Autodesk Inventor part; units mm, degrees
ref_plane "YZ Plane" through (0, 0, 0) normal (1, 0, 0) x (0, 1, 0)
ref_plane "XZ Plane" through (0, 0, 0) normal (0, 1, 0) x (-1, 0, 0)
ref_plane "XY Plane" through (0, 0, 0) normal (0, 0, 1) x (1, 0, 0)
sketch "Sketch1" plane through (0, 0, 0) normal (0, 1, 0) x (-1, 0, 0)
  line L0 (-83.5, 139.5) -> (83.5, 139.5)
  line L1 (83.5, 139.5) -> (83.5, -139.5)
  line L2 (83.5, -139.5) -> (-83.5, -139.5)
  line L3 (-83.5, -139.5) -> (-83.5, 139.5)
  line L4 (-83.5, 139.5) -> (83.5, -139.5) construction
  line L5 (83.5, 139.5) -> (-83.5, -139.5) construction
  point P0 (0, 0)
  dimension "d0" = 167
  dimension "d1" = 279
extrude "Extrusion1" add sketch "Sketch1" along normal blind 26.6
sketch "Sketch2" plane through (0, 26.6, 0) normal (0, 1, 0) x (1, 0, 0)
  line L0 (71.5, -119.5) -> (-71.5, -119.5)
  line L1 (-73.5, -117.5) -> (-73.5, 117.5)
  line L2 (-71.5, 119.5) -> (71.5, 119.5)
  line L3 (73.5, 117.5) -> (73.5, -117.5)
  line L4 (73.5, -119.5) -> (-73.5, 119.5) construction
  line L5 (-73.5, -119.5) -> (73.5, 119.5) construction
  arc A0 (-73.5, -117.5) -> (-71.5, -119.5) centre (-71.5, -117.5) ccw
  arc A1 (-71.5, 119.5) -> (-73.5, 117.5) centre (-71.5, 117.5) ccw
  arc A2 (73.5, 117.5) -> (71.5, 119.5) centre (71.5, 117.5) ccw
  arc A3 (71.5, -119.5) -> (73.5, -117.5) centre (71.5, -117.5) ccw
  point P0 (0, 0)
  dimension "d4" = 147
  dimension "d5" = 239
  dimension "d6" = 2
extrude "Extrusion2" cut sketch "Sketch2" against normal blind 1.1
sketch "Sketch3" plane through (0, 25.5, 0) normal (0, 1, 0) x (1, 0, 0)
  line L0 (-73.5, -117.5) -> (-73.5, 117.5)
  line L1 (71.5, -119.5) -> (-71.5, -119.5)
  line L2 (-72.25, -117.83) -> (72.25, -117.83)
  line L3 (72.25, -117.83) -> (72.25, 112.27)
  line L4 (72.25, 112.27) -> (-72.25, 112.27)
  line L5 (-72.25, 112.27) -> (-72.25, -117.83)
  point P0 (0, 0)
  dimension "d9" = 1.25
  dimension "d10" = 1.67
  dimension "d11" = 144.5
  dimension "d12" = 230.1
extrude "Extrusion3" cut sketch "Sketch3" against normal blind 20
sketch "Sketch4" plane through (0, 5.5, 0) normal (0, 1, 0) x (1, 0, 0)
  circle A0 centre (-66.5, -111.83) radius 2
  line L0 (72.25, -117.83) -> (-72.25, -117.83)
  line L1 (-72.25, -117.83) -> (-72.25, 112.27)
  circle A1 centre (66.5, -111.83) radius 2
  line L2 (72.25, 112.27) -> (72.25, -117.83)
  circle A2 centre (-66.5, 106.27) radius 2
  line L3 (-72.25, 112.27) -> (72.25, 112.27)
  circle A3 centre (66.5, 106.27) radius 2
  point P0 (0, 0)
  dimension "d15" = 4
  dimension "d16" = 6
  dimension "d17" = 5.75
  dimension "d18" = 4
  dimension "d19" = 6
  dimension "d20" = 5.75
  dimension "d21" = 4
  dimension "d22" = 5.75
  dimension "d23" = 6
  dimension "d24" = 4
  dimension "d25" = 6
  dimension "d26" = 5.75
extrude "Extrusion4" add sketch "Sketch4" along normal blind 10.3 contours A0 | A1 | A2 | A3
sketch "Sketch5" plane through (0, 5.5, 0) normal (0, 1, 0) x (1, 0, 0)
  circle A0 centre (-66.5, -111.83) radius 2
  circle A1 centre (-66.5, -111.83) radius 1.25
  circle A2 centre (-66.5, 106.27) radius 2
  circle A3 centre (-66.5, 106.27) radius 1.25
  circle A4 centre (66.5, 106.27) radius 2
  circle A5 centre (66.5, 106.27) radius 1.25
  circle A6 centre (66.5, -111.83) radius 1.25
  point P0 (0, 0)
  dimension "d29" = 2.5
  dimension "d30" = 2.5
  dimension "d31" = 2.5
  dimension "d32" = 2.5
extrude "Extrusion5" cut sketch "Sketch5" along normal blind 10.3 and the other way blind 5.5 contours A1 | A3 | A5 | A6
sketch "Sketch8" plane through (0, 0, 0) normal (0, -1, 0) x (1, 0, 0)
  circle A0 centre (66.5, 111.83) radius 1.25
  circle A1 centre (66.5, 111.83) radius 1.75
  circle A2 centre (66.5, -106.27) radius 1.25
  circle A3 centre (66.5, -106.27) radius 1.75
  circle A4 centre (-66.5, -106.27) radius 1.25
  circle A5 centre (-66.5, -106.27) radius 1.75
  circle A6 centre (-66.5, 111.83) radius 1.75
  point P0 (0, 0)
  dimension "d49" = 3.5
  dimension "d50" = 3.5
  dimension "d51" = 3.5
  dimension "d52" = 3.5
extrude "Extrusion8" cut sketch "Sketch8" against normal blind 13.8
sketch "Sketch9" plane through (0, 5.5, 0) normal (0, 1, 0) x (1, 0, 0)
  line L0 (60, -100) -> (-60, -100)
  line L1 (-60, -100) -> (-60, 100)
  line L2 (-60, 100) -> (60, 100)
  line L3 (60, 100) -> (60, -100)
  line L4 (60, -100) -> (-60, 100) construction
  line L5 (-60, -100) -> (60, 100) construction
  point P0 (0, 0)
  dimension "d55" = 120
  dimension "d56" = 200
extrude "Extrusion9" cut sketch "Sketch9" against normal blind 5.8
sketch "Sketch10" plane through (0, 0, 0) normal (0, -1, 0) x (1, 0, 0)
  line L0 (83.5, 139.5) -> (83.5, -139.5)
  line L1 (-83.5, -139.5) -> (-83.5, 139.5)
  line L2 (83.5, 139.5) -> (-83.5, 139.5)
  line L3 (-83.5, 139.5) -> (-83.5, -139.5)
  line L4 (-83.5, -139.5) -> (83.5, -139.5)
  line L5 (83.5, -139.5) -> (83.5, 139.5)
  line L6 (72.25, -115.05) -> (-72.25, -115.05)
  line L7 (-72.25, -115.05) -> (-72.25, 115.05)
  line L8 (-72.25, 115.05) -> (72.25, 115.05)
  line L9 (72.25, 115.05) -> (72.25, -115.05)
  line L10 (72.25, -115.05) -> (-72.25, 115.05) construction
  line L11 (-72.25, -115.05) -> (72.25, 115.05) construction
  line L12 (-83.5, -139.5) -> (83.5, -139.5)
  line L13 (83.5, -139.5) -> (83.5, 139.5)
  line L14 (83.5, 139.5) -> (-83.5, 139.5)
  line L15 (-83.5, 139.5) -> (-83.5, -139.5)
  point P0 (0, 0)
  point P1 (71.5, 119.5)
  dimension "d67" = 144.5
  dimension "d68" = 230.1
extrude "Extrusion10" add sketch "Sketch10" along normal blind 40
sketch "Sketch12" plane through (0, -40, 0) normal (0, -1, 0) x (1, 0, 0)
  line L0 (-72.25, -115.05) -> (-72.25, 115.05)
  line L1 (72.25, -115.05) -> (-72.25, -115.05)
  line L2 (-77.25, -120.05) -> (-72.25, -120.05)
  line L3 (-72.25, -120.05) -> (-72.25, 120.05)
  line L4 (-72.25, 120.05) -> (-77.25, 120.05)
  line L5 (-77.25, 120.05) -> (-77.25, -120.05)
  line L6 (72.25, 115.05) -> (72.25, -115.05)
  line L7 (77.25, -120.05) -> (72.25, -120.05)
  line L8 (72.25, -120.05) -> (72.25, 120.05)
  line L9 (72.25, 120.05) -> (77.25, 120.05)
  line L10 (77.25, 120.05) -> (77.25, -120.05)
  line L11 (72.25, 115.05) -> (-72.25, 115.05)
  line L12 (72.25, 120.05) -> (-72.25, 120.05)
  line L13 (-72.25, 120.05) -> (-72.25, 115.05)
  line L14 (-72.25, 115.05) -> (72.25, 115.05)
  line L15 (72.25, 115.05) -> (72.25, 120.05)
  line L16 (-83.5, 139.5) -> (-83.5, -139.5)
  line L17 (83.5, 139.5) -> (-83.5, 139.5)
  line L18 (-83.5, -139.5) -> (83.5, -139.5)
  line L19 (83.5, -139.5) -> (83.5, 139.5)
  line L20 (83.5, 139.5) -> (-83.5, 139.5)
  line L21 (-83.5, 139.5) -> (-83.5, -139.5)
  line L22 (-72.25, -115.05) -> (72.25, -115.05)
  line L23 (-72.25, -115.05) -> (72.25, -115.05)
  line L24 (72.25, -115.05) -> (72.25, -120.05)
  line L25 (72.25, -120.05) -> (-72.25, -120.05)
  line L26 (-72.25, -120.05) -> (-72.25, -115.05)
  point P0 (0, 0)
  dimension "d69" = 5
  dimension "d70" = 5
  dimension "d71" = 240.1
  dimension "d72" = 5
  dimension "d73" = 5
  dimension "d74" = 240.1
extrude "Extrusion11" add sketch "Sketch12" along normal blind 10
sketch "Sketch13" plane through (0, -50, 0) normal (0, -1, 0) x (1, 0, 0)
  circle A0 centre (-77.5, -133.5) radius 1.25
  line L0 (-83.5, 139.5) -> (-83.5, -139.5)
  line L1 (-83.5, -139.5) -> (83.5, -139.5)
  circle A1 centre (-77.5, 133.5) radius 1.25
  line L2 (83.5, 139.5) -> (-83.5, 139.5)
  circle A2 centre (77.5, 133.5) radius 1.25
  line L3 (83.5, -139.5) -> (83.5, 139.5)
  circle A3 centre (77.5, -133.5) radius 1.25
  point P0 (0, 0)
  dimension "d77" = 2.5
  dimension "d78" = 6
  dimension "d79" = 6
  dimension "d80" = 2.5
  dimension "d81" = 6
  dimension "d82" = 6
  dimension "d83" = 2.5
  dimension "d84" = 6
  dimension "d85" = 6
  dimension "d86" = 6
  dimension "d87" = 6
extrude "Extrusion12" cut sketch "Sketch13" against normal blind 10 contours A0 | A1 | A2 | A3
sketch "Sketch14" plane through (83.5, 26.6, 139.5) normal (1, 0, 0) x (0, 0, -1)
  line L0 (0, 0) -> (279, 0)
  line L1 (139.5, 0) -> (139.5, -76.6)
  line L2 (259.55, -76.6) -> (19.45, -76.6)
  point P0 (139.5, -26.6)
split_face "Split1"
sketch "Sketch16" plane through (83.5, -50, 0) normal (1, 0, 0) x (0, 0, -1)
  line L0 (-139.5, 0) -> (-139.5, 76.6)
  line L1 (-139.5, 76.6) -> (0, 76.6)
  line L2 (0, 76.6) -> (0, 0)
  line L3 (0, 0) -> (-139.5, 0)
  line L4 (-139.5, 0) -> (-139.5, 76.6)
  point P0 (0, 50)
extrude "Extrusion13" cut sketch "Sketch16" against normal blind 167.1625
sketch "Sketch17" plane through (-72.25, 0, 0) normal (0, 0, 1) x (1, 0, 0)
  circle A0 centre (-6.25, 16) radius 2.5
  circle A1 centre (-6.25, -4) radius 2.5
  circle A2 centre (-6.25, -24) radius 2.5
  line L0 (155.75, 26.6) -> (145.75, 26.6)
  circle A3 centre (150.75, 16) radius 2.5
  circle A4 centre (150.75, -4) radius 2.5
  circle A5 centre (150.75, -24) radius 2.5
  point P0 (72.25, 0)
  dimension "d92" = 5
  dimension "d95" = 5
  dimension "d97" = 5
  dimension "d99" = 5
extrude "Extrusion14" add sketch "Sketch17" along normal blind 15
properties part number "Enclosure"
Can you work these out from the model? Positions are in its coordinate system, mm. A direction names the side the tool comes from. Give positions to 0.01 mm unless a question says otherwise; leave off trailing zeros. Loops run counter-clockwise (first coordinate to the right, second up) from the corner with the lowest first, then second, coordinate; pieces in that order, holes last. Notation, with made-up numbers: M 6.25,15 L 34.25,15 A20 cw 34.25,23 Z; hole C 0.5,60.25 d10. An arc over 180 degrees is marked long. Answer in a Markdown table with one row per item.
1. Suppose I cut it at A-A on y = 10.5. Write out the boundary of the cut face in (x, z), plus the area to 3 significant figures.
Taken from the geometry:
| item | result |
|---|---|
| outline | M -83.5,-139.5 L 83.5,-139.5 L 83.5,0 L 72.25,0 L 72.25,-112.27 L -72.25,-112.27 L -72.25,0 L -83.5,0 Z; C -66.5,-106.27 d4; C 66.5,-106.27 d4; hole C -66.5,-106.27 d3.5; hole C 66.5,-106.27 d3.5 |
| area | 7,080 mm² |
2. Thinking about a two-plate mould opening in X: for faces 1 (the flat face through (-5, 0, -104)), 2 (the flat face through (78, 16, 15)), 3 (the flat face through (83.5, -11, -71)), which applies, released by +X, released by -X, zero draft, split by the parting line, or undercut?
Taken from the geometry:
| item | result |
|---|---|
| face 1 | undercut |
| face 2 | zero draft |
| face 3 | released by +X |
3. If I drill on line 1 along X through (y, z) = (14.3, -106.27); line 2 along X through (y, z) = (6, -106.27); line 3 along Z through (x, y) = (-66.5, 7), over which ranges is the centre line in solid material (lowest first)?
Taken from the geometry:
| item | result |
|---|---|
| line 1 | x = -83.5 to -72.25, -68.5 to -67.75, -65.25 to -64.5, 64.5 to 65.25, 67.75 to 68.5, 72.25 to 83.5 |
| line 2 | x = -83.5 to -72.25, -68.5 to -68.25, -64.75 to -64.5, 64.5 to 64.75, 68.25 to 68.5, 72.25 to 83.5 |
| line 3 | z = -139.5 to -112.27, -108.27 to -108.02, -104.52 to -104.27 |
4. Suppose I cut it at D-D on y = -24. Write out the boundary of the cut face in (x, z), plus the area to 3 significant figures.
Taken from the geometry:
| item | result |
|---|---|
| outline | M -83.5,-139.5 L 83.5,-139.5 L 83.5,0 L 81,0 L 81,15 L 76,15 L 76,0 L 72.25,0 L 72.25,-115.05 L -72.25,-115.05 L -72.25,0 L -76,0 L -76,15 L -81,15 L -81,0 L -83.5,0 Z |
| area | 6,820 mm² |
5. Suppose I cut it at C-C on y = -9. Write out the boundary of the cut face in (x, z), plus the area to 3 significant figures.
Taken from the geometry:
| item | result |
|---|---|
| outline | M -83.5,-139.5 L 83.5,-139.5 L 83.5,0 L 72.25,0 L 72.25,-115.05 L -72.25,-115.05 L -72.25,0 L -83.5,0 Z |
| area | 6,670 mm² |
6. Suppose I cut it at B-B on z = -55. Write out the boundary of the cut face in (x, y), plus the area to 3 significant figures.
Taken from the geometry:
| item | result |
|---|---|
| outline | M -83.5,-50 L -77.25,-50 L -77.25,-40 L -72.25,-40 L -72.25,0 L -60,0 L -60,5.5 L -72.25,5.5 L -72.25,25.5 L -73.5,25.5 L -73.5,26.6 L -83.5,26.6 Z; M 60,0 L 72.25,0 L 72.25,-40 L 77.25,-40 L 77.25,-50 L 83.5,-50 L 83.5,26.6 L 73.5,26.6 L 73.5,25.5 L 72.25,25.5 L 72.25,5.5 L 60,5.5 Z |
| area | 1,760 mm² |
7. For pin 1 Ø1.8 at (x, z) = (-66, -106) entering from -Y; pin 2 Ø3 at (x, z) = (66.5, -106.27) entering from +Y; pin 3 Ø3 at (x, y) = (20, 2) entering from +Z, each with a flat end and sliding along its axis, tell me the tip position at first contact or that it passes through.
Taken from the geometry:
| item | result |
|---|---|
| pin 1 | stops at y = 13.8 |
| pin 2 | stops at y = 15.8 |
| pin 3 | stops at z = -100 |
8. Which directions (+Z, -Z, +X, -X, +Y, -Y) give clear straight access to the entire face, cutting with the end or side of a thin tool? Please do faces 4 (the cylindrical face through (76, -4, 7)), 5 (the cylindrical face through (66.066, 10.578, -108.222)), 6 (the flat face through (60, 3, -51)), 7 (the flat face through (72.25, -20, -57)), 8 (the flat face through (68, 15.8, -106)).
Taken from the geometry:
| item | result |
|---|---|
| face 4 | +Z |
| face 5 | +Y |
| face 6 | +Z, +Y, -Y |
| face 7 | +Z, -Y |
| face 8 | +Z, +Y |
